from build123d import *

# Parameters (mm, degrees)
SKETCH1_R           = 248.894047882
SKETCH1_R_2         = 4
BOSS_EXTRUDE1_DEPTH = 1.5875


with BuildPart() as part:
    # Sketch1 → Boss-Extrude1 (new, symmetric)
    with BuildSketch(Plane(origin=(0, 79.166310833, -2.766864901), x_dir=(0, -0.03492870325036397, -0.9993898066766781), z_dir=(0, -0.9993898066766781, 0.03492870325036397))):
        with Locations((28.500583785, 0)):
            Circle(SKETCH1_R)
        with Locations((-119.119809099, 0)):
            Circle(SKETCH1_R_2, mode=Mode.SUBTRACT)
        with Locations((126.54316519, -59)):
            Circle(SKETCH1_R_2, mode=Mode.SUBTRACT)
        with Locations((126.54316519, 59)):
            Circle(SKETCH1_R_2, mode=Mode.SUBTRACT)
        with BuildLine():
            ThreePointArc((238.081851524, -78.766978422), (252.394631667, 0), (238.081851524, 78.766978422))
            ThreePointArc((238.081851524, 78.766978422), (233.209259095, 84.18518249), (225.953504109, 84.858318353))
            ThreePointArc((225.953504109, 84.858318353), (143.037826046, 53.222841583), (66.585433619, 8.157946694))
            ThreePointArc((66.585433619, 8.157946694), (62.36885006, 0), (66.585433619, -8.157946694))
            ThreePointArc((66.585433619, -8.157946694), (143.037826046, -53.222841583), (225.953504109, -84.858318353))
            ThreePointArc((225.953504109, -84.858318353), (233.209259095, -84.18518249), (238.081851524, -78.766978422))
        make_face(mode=Mode.SUBTRACT)
        with BuildLine():
            ThreePointArc((-184.986589143, 16.62098717), (-96.058103224, 13.003455955), (-7.783793413, 24.361640995))
            ThreePointArc((-7.783793413, 24.361640995), (-1.152695169, 29.274262086), (-0.472616045, 37.498786528))
            ThreePointArc((-0.472616045, 37.498786528), (-35.031535638, 114.339868269), (-81.363716284, 184.71173625))
            ThreePointArc((-81.363716284, 184.71173625), (-87.629404707, 188.431983672), (-94.756155234, 186.912602473))
            ThreePointArc((-94.756155234, 186.912602473), (-161.65529586, 118.191734539), (-193.66286294, 27.783945296))
            ThreePointArc((-193.66286294, 27.783945296), (-191.635746069, 20.406253949), (-184.986589143, 16.62098717))
        make_face(mode=Mode.SUBTRACT)
        with BuildLine():
            ThreePointArc((-184.986589143, -16.62098717), (-96.058103224, -13.003455955), (-7.783793413, -24.361640995))
            ThreePointArc((-7.783793413, -24.361640995), (-1.152695169, -29.274262086), (-0.472616045, -37.498786528))
            ThreePointArc((-0.472616045, -37.498786528), (-35.031535638, -114.339868269), (-81.363716284, -184.71173625))
            ThreePointArc((-81.363716284, -184.71173625), (-87.629404707, -188.431983672), (-94.756155234, -186.912602473))
            ThreePointArc((-94.756155234, -186.912602473), (-161.65529586, -118.191734539), (-193.66286294, -27.783945296))
            ThreePointArc((-193.66286294, -27.783945296), (-191.635746069, -20.406253949), (-184.986589143, -16.62098717))
        make_face(mode=Mode.SUBTRACT)
        with BuildLine():
            ThreePointArc((205.754686462, 136.78277582), (122.671836524, 203.126364203), (18.352909122, 223.663965305))
            ThreePointArc((18.352909122, 223.663965305), (11.694176969, 220.704171659), (8.811835123, 214.01154902))
            ThreePointArc((8.811835123, 214.01154902), (12.86563705, 128.486999921), (30.677726566, 44.739693841))
            ThreePointArc((30.677726566, 44.739693841), (35.60655975, 38.753388876), (43.332423143, 38.089854005))
            ThreePointArc((43.332423143, 38.089854005), (127.305687629, 73.474816574), (203.951454434, 122.760018767))
            ThreePointArc((203.951454434, 122.760018767), (207.756142558, 129.39808179), (205.754686462, 136.78277582))
        make_face(mode=Mode.SUBTRACT)
        with BuildLine():
            ThreePointArc((8.811835123, -214.01154902), (12.86563705, -128.486999921), (30.677726566, -44.739693841))
            ThreePointArc((30.677726566, -44.739693841), (35.60655975, -38.753388876), (43.332423143, -38.089854005))
            ThreePointArc((43.332423143, -38.089854005), (127.305687629, -73.474816574), (203.951454434, -122.760018767))
            ThreePointArc((203.951454434, -122.760018767), (207.756142558, -129.39808179), (205.754686462, -136.78277582))
            ThreePointArc((205.754686462, -136.78277582), (122.671836524, -203.126364203), (18.352909122, -223.663965305))
            ThreePointArc((18.352909122, -223.663965305), (11.694176969, -220.704171659), (8.811835123, -214.01154902))
        make_face(mode=Mode.SUBTRACT)
        with BuildLine():
            ThreePointArc((-52.210070583, -208.840453333), (-40.68648195, -212.935893198), (-28.956463756, -216.3960082))
            ThreePointArc((-28.956463756, -216.3960082), (-20.219684914, -214.600125685), (-16.391954321, -206.543763165))
            ThreePointArc((-16.391954321, -206.543763165), (-16.412181984, -186.973684298), (-15.74049523, -167.415125227))
            ThreePointArc((-15.74049523, -167.415125227), (-22.636803093, -157.38469373), (-34.111773062, -161.445935215))
            ThreePointArc((-34.111773062, -161.445935215), (-45.06459964, -177.663949457), (-56.583967908, -193.484586319))
            ThreePointArc((-56.583967908, -193.484586319), (-58.222679885, -202.252204103), (-52.210070583, -208.840453333))
        make_face(mode=Mode.SUBTRACT)
        with BuildLine():
            ThreePointArc((-16.391954321, 206.543763165), (-16.412181984, 186.973684298), (-15.74049523, 167.415125227))
            ThreePointArc((-15.74049523, 167.415125227), (-22.636803093, 157.38469373), (-34.111773062, 161.445935215))
            ThreePointArc((-34.111773062, 161.445935215), (-45.06459964, 177.663949457), (-56.583967908, 193.484586319))
            ThreePointArc((-56.583967908, 193.484586319), (-58.222679885, 202.252204103), (-52.210070583, 208.840453333))
            ThreePointArc((-52.210070583, 208.840453333), (-40.68648195, 212.935893198), (-28.956463756, 216.3960082))
            ThreePointArc((-28.956463756, 216.3960082), (-20.219684914, 214.600125685), (-16.391954321, 206.543763165))
        make_face(mode=Mode.SUBTRACT)
    extrude(amount=BOSS_EXTRUDE1_DEPTH, both=True)


solid = part.part
Geometry check sheet. Reference: the model listing, model coordinates, mm. Give positions to 0.01 mm unless a question says otherwise; leave off trailing zeros. Loops run counter-clockwise (first coordinate to the right, second up) from the corner with the lowest first, then second, coordinate; pieces in that order, holes last.
(1) Thickness scan on L1, parallel to X at y = 73.75, z = -146; L2, parallel to X at y = 83.5, z = 79.5; L3, parallel to X at y = 71.5, z = -206. Record the ranges inside material, lowest first.
From the geometry:
L1: x = -220.82 to -192.2, -82.28 to -53.37, 53.37 to 82.28, 192.2 to 220.82
L2: x = -222.84 to -185.82, -13.78 to 13.78, 185.82 to 222.84
L3: x = -177.11 to -139.81, -122.32 to -77.81, 77.81 to 122.32, 139.81 to 177.11
(2) Depth check by flat-ended pin: pin 1 Ø12 at (x, z) = (164, 32) entering from +Y; pin 2 Ø3 at (x, y) = (-90, 78) entering from +Z; pin 3 Ø10 at (x, z) = (-184, -202) entering from +Y. Enter the tip coordinate at first touch or a pass-through.
From the geometry:
pin 1: stops at y = 82.18
pin 2: stops at z = 20.45
pin 3: stops at y = 73.97
(3) Section check B-B on x = 173.5. Record the cut outline in (y, z), then the cut area to 3 significant figures.
From the geometry:
outline: (70.35, -209.54) - (73.52, -209.65) - (74.81, -172.73) - (71.64, -172.62) - close; (77.27, -11.7) - (80.44, -11.82) - (81.31, 13.19) - (78.14, 13.3) - close; (79.05, 39.44) - (82.23, 39.32) - (83.3, 70) - (80.12, 70.11) - close; (81.53, 110.23) - (84.7, 110.12) - (85.99, 147.04) - (82.82, 147.15) - close
area: 411 mm2
(4) Section check C-C on z = 128. Count the separate pieces of the cut face and the enclosed holes in it, then the cut area to 3 significant figures.
From the geometry:
separate pieces: 3
enclosed holes: 0
area: 296 mm2
(5) Section check A-A on x = 110. Record the cut outline in (y, z).
From the geometry:
outline: (68.79, -254.33) - (71.96, -254.44) - (74.23, -189.43) - (71.06, -189.32) - close; (77.04, -18.29) - (80.21, -18.4) - (81.89, 29.83) - (78.72, 29.94) - close; (83.4, 163.7) - (86.57, 163.58) - (87.56, 191.83) - (84.38, 191.94) - close
